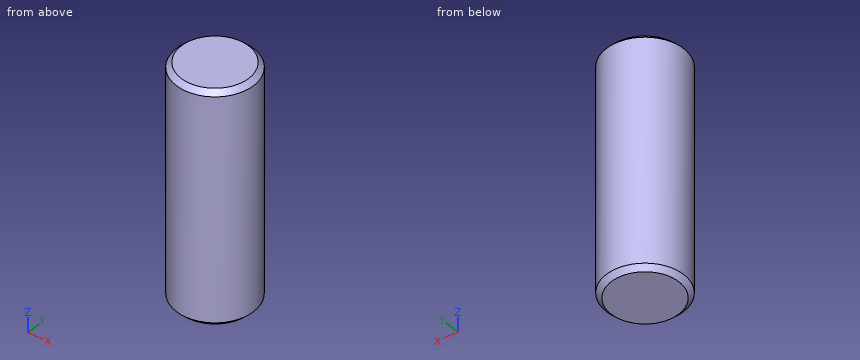
Autodesk Inventor part; units mm, degrees
ref_plane "YZ Plane" through (0, 0, 0) normal (1, 0, 0) x (0, 1, 0)
ref_plane "XZ Plane" through (0, 0, 0) normal (0, 1, 0) x (-1, 0, 0)
ref_plane "XY Plane" through (0, 0, 0) normal (0, 0, 1) x (1, 0, 0)
sketch "Sketch1" plane through (0, 0, 0) normal (0, 0, 1) x (1, 0, 0)
  line L0 (-11.2, 0) -> (11.2, 0)
  line L1 (0, -11.2) -> (0, 11.2)
  circle A0 centre (0, 0) radius 8
  dimension "d0" = 8
extrude "Extrusion1" add sketch "Sketch1" along normal blind 48
chamfer "Chamfer1" distance 1 angle 45 1 edges at (-8, 0, 48)
chamfer "Chamfer2" distance 1 angle 45 1 edges at (-8, 0, 0)
properties part number "Ax"
Check sheet for the modelled part. Datum: model origin and axes. Units: mm. Round coordinates to 2 decimals unless told otherwise and drop trailing zeros. Loops run counter-clockwise (first coordinate to the right, second up) from the corner with the lowest first, then second, coordinate; pieces in that order, holes last. Notation, with made-up numbers: (-24.5, -35) - (-15.5, -35) arc R19 cw to (-15.5, -20) - close; hole circle Ø2 at (77.5, 61). An arc over 180 degrees is marked (long way). Answer as a JSON object with one key per item and string values. Group by question number.
Q1. Scan lines: line 1 along X through (y, z) = (-0.25, 43); line 2 along X through (y, z) = (-2, 6); line 3 along Y through (x, z) = (6, 19). Record each from-to range of solid material in increasing order. Write a range as [from, to].
Q2. Sectioned sample at A-A, the plane z = 16.5. Enter the section's corners in (x, y).
Q3. Gauge pin test, flat ends, axial feed: P1, Ø4, axis at y = -0.5, z = 12.5, coming from the -X side; P2, Ø3, axis at y = -4, z = 34, coming from the -X side; P3, Ø1.5, axis at y = 4.5, z = 29, coming from the +X side; P4, Ø1, axis at x = 5.5, z = 41.5, coming from the -Y side (3 decimals). Record the tip position at first contact, or that the pin passes through.
Solution:
{
 "1": {"line 1": "x = [-8, 8]", "line 2": "x = [-7.75, 7.75]", "line 3": "y = [-5.29, 5.29]"},
 "2": {"outline": "circle Ø16 at (0, 0)"},
 "3": {"P1": "stops at x = -8", "P2": "stops at x = -7.6", "P3": "stops at x = 7.07", "P4": "stops at y = -6.245"}
}
